```python
from build123d import *

# Parameters (mm, degrees)
F0_W     = 95.25
F0_H     = 41.275
F1_DEPTH = 203.2
F2_SIZE  = 41.27499


# Not quite as in the source:
# - a fillet or chamfer is up to 0.001 mm smaller than in the source, because OpenCascade refuses the exact size


with BuildPart() as f1:
    # F0 (on Right) → F1 (new body)
    with BuildSketch(Plane.YZ):
        Rectangle(F0_W, F0_H)
    extrude(amount=-F1_DEPTH)

    # F2 (size 41.275 in the source; OpenCascade refuses exactly that, so slightly less here)
    f2_edges = [f1.edges().sort_by_distance(p)[0] for p in [
        (-101.6, -47.625, 20.6375),
        (-101.6, 47.625, 20.6375),
    ]]
    chamfer(f2_edges, length=F2_SIZE)


solid = f1.part
```
The listing builds one solid part. Answer for the finished solid, in the listing's coordinates (mm). Round coordinates to 2 decimals unless told otherwise and drop trailing zeros. Loops run counter-clockwise (first coordinate to the right, second up) from the corner with the lowest first, then second, coordinate; pieces in that order, holes last. Notation, with made-up numbers: (88, -21) -> (137, -21) arc R24 ccw to (137, -2) -> close; hole circle Ø8 at (62.5, -17.5). An arc over 180 degrees is marked (long way). Use one line per item in the form item = value.
1. The part is cut by section B-B on y = -14.5. Determine the outline of the cut face in (x, z), and give its area (3 significant figures).
Answer key:
outline = (-203.2, -20.64) -> (0, -20.64) -> (0, 12.49) -> (-203.2, 12.49) -> close
area = 6,730 mm²
2. Flat-ended cylindrical pins translate along their axes: pin 1 Ø5 at (x, z) = (-48.5, 14.5) entering from +Y; pin 2 Ø6 at (x, y) = (-152.5, -34.5) entering from +Z; pin 3 Ø1 at (x, z) = (-167.5, -0.5) entering from +Y; pin 4 Ø8 at (x, y) = (-69, 6.5) entering from +Z. Find the tip coordinate at first contact, or state that the pin passes through.
Answer key:
pin_1 = 14.99
pin_2 = -4.51
pin_3 = 27.99
pin_4 = 20.64
3. The part is cut by section C-C on z = 17.5. Determine the outline of the cut face in (x, y).
Answer key:
outline = (-203.2, -9.49) -> (0, -9.49) -> (0, 9.49) -> (-203.2, 9.49) -> close
4. Find the intervals of material crossed by probe 1 along Y at (x, z) = (-48, 19); probe 2 along Z at (x, y) = (-190, 26.5); probe 3 along Z at (x, y) = (-26, 11.5), in increasing order. Write a range as [from, to].
Answer key:
probe_1 = [-7.99, 7.99]
probe_2 = [-20.64, 0.49]
probe_3 = [-20.64, 15.49]
